Answer from the drawing. Dimensions are ordinates in mm from the lowest x, y and z of the part. Coordinates: 2 decimals unless noted, no trailing zeros. Write each loop counter-clockwise with the first axis right and the second up, starting at its lowest first coordinate (ties: lowest second). Pieces come first, ordered by that corner, then holes. Notation, with made-up numbers: (-38, 51.5) -> (9, 51.5) arc R14 cw to (9, 59.5) -> close; hole circle Ø8 at (81.5, -12). An arc over 180 degrees is marked (long way). Use CSV: the item, a comma, the result in double quotes.
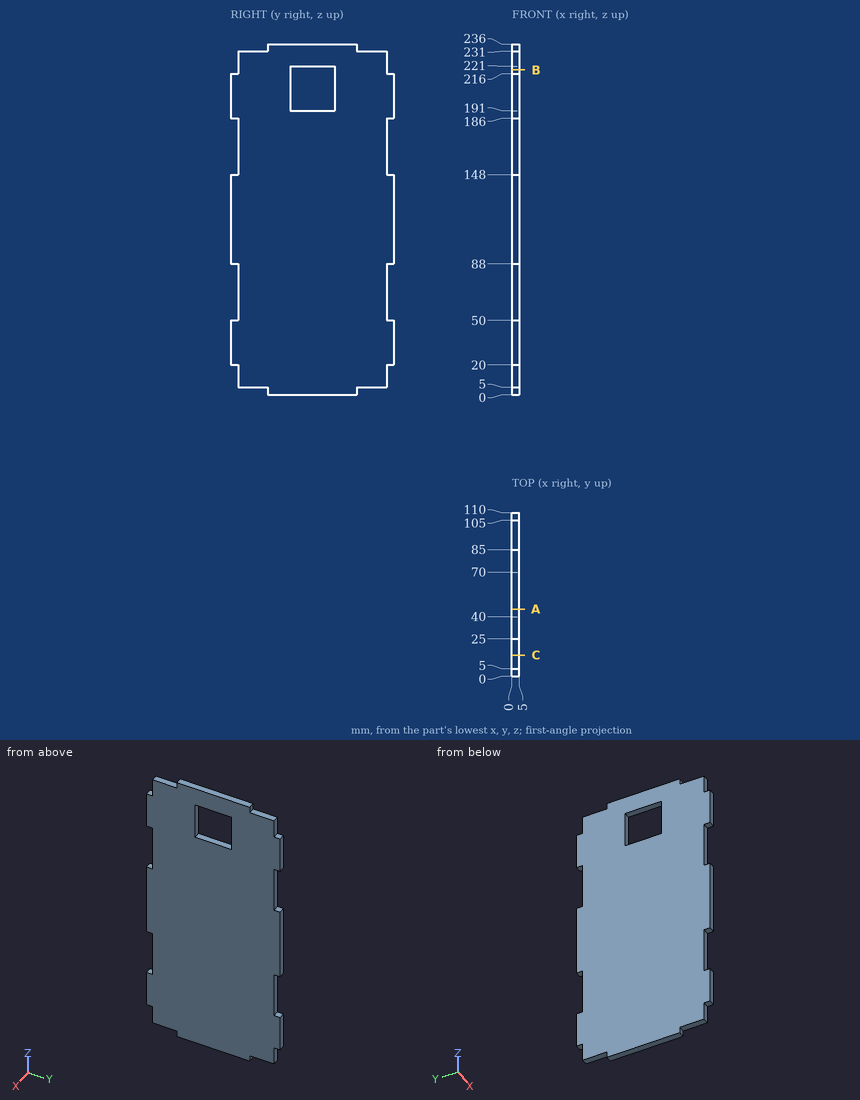
1. A cutting plane is placed at C-C (y = 14). Give the vertices of the cut face in (x, z), and give its area (3 significant figures).
Solutions:
outline,"(0, 5) -> (5, 5) -> (5, 231) -> (0, 231) -> close"
area,"1,130 mm^2"
2. A cutting plane is placed at B-B (z = 218.5). Give the vertices of the cut face in (x, y).
Solutions:
outline,"(0, 5) -> (5, 5) -> (5, 40) -> (0, 40) -> close; (0, 70) -> (5, 70) -> (5, 105) -> (0, 105) -> close"
3. A cutting plane is placed at A-A (y = 45). Give the vertices of the cut face in (x, z), and give its area (3 significant figures).
Solutions:
outline,"(0, 0) -> (5, 0) -> (5, 191) -> (0, 191) -> close; (0, 221) -> (5, 221) -> (5, 236) -> (0, 236) -> close"
area,"1,030 mm^2"
4. Find the intervals of material crossed by line 1 along Z through (x, y) = (0.9, 105.5); line 2 along Z through (x, y) = (0.95, 46); line 3 along Y through (x, z) = (2.15, 73.5), in increasing order.
Solutions:
line 1,"z = 20 to 50, 88 to 148, 186 to 216"
line 2,"z = 0 to 191, 221 to 236"
line 3,"y = 5 to 105"
5. Each of these flat-tipped pins is pushed along its axis until it touches: pin 1 Ø4 at (y, z) = (94.5, 67.5) entering from -X; pin 2 Ø2.5 at (x, y) = (1.5, 3) entering from -Z; pin 3 Ø2.5 at (x, z) = (2, 226.5) entering from -Y; pin 4 Ø2.5 at (x, z) = (3, 9.5) entering from +Y. Where does it stop, or does it pass through?
Solutions:
pin 1,"stops at x = 0"
pin 2,"stops at z = 20"
pin 3,"stops at y = 5"
pin 4,"stops at y = 105"
